Can you work these out from the model? Positions are in its coordinate system, mm. Face numbers are marked on the shaded views. A direction names the side the tool comes from. Give positions to 0.01 mm unless a question says otherwise; leave off trailing zeros. Loops run counter-clockwise (first coordinate to the right, second up) from the corner with the lowest first, then second, coordinate; pieces in that order, holes last. Notation, with made-up numbers: M 1.25,-17 L 17.25,-17 A6 ccw 17.25,-7 Z; hole C -10,44 d4. An arc over 180 degrees is marked long. Answer as a JSON object with one key per item and string values.
Autodesk Inventor part; units mm, degrees
ref_plane "Work Plane1" through (0, 0, 15) normal (0, 0, -1) x (-1, 0, 0)
ref_plane "YZ Plane" through (0, 0, 0) normal (1, 0, 0) x (0, 1, 0)
ref_plane "XZ Plane" through (0, 0, 0) normal (0, 1, 0) x (-1, 0, 0)
sketch "Sketch1" plane through (0, 0, 0) normal (0, 0, 1) x (1, 0, 0)
  line L0 (-12.5, 12.5) -> (12.5, 12.5) construction
  line L1 (12.5, 12.5) -> (12.5, -12.5) construction
  line L2 (12.5, -12.5) -> (-12.5, -12.5) construction
  line L3 (-12.5, -12.5) -> (-12.5, 12.5) construction
  line L4 (-12.5, 12.5) -> (12.5, -12.5) construction
  line L5 (12.5, 12.5) -> (-12.5, -12.5) construction
  circle A0 centre (-12.5, 12.5) radius 3
  circle A1 centre (12.5, 12.5) radius 3
  circle A2 centre (12.5, -12.5) radius 3
  circle A3 centre (-12.5, -12.5) radius 3
  line L6 (-18.5, -18.5) -> (18.5, -18.5)
  line L7 (18.5, -18.5) -> (18.5, -6.5)
  line L8 (18.5, -6.5) -> (-18.5, -6.5)
  line L9 (-18.5, -6.5) -> (-18.5, -18.5)
  line L10 (-18.5, -18.5) -> (18.5, -6.5) construction
  line L11 (18.5, -18.5) -> (-18.5, -6.5) construction
  point P0 (0, 0)
  point P1 (0, -12.5)
  dimension "d0" = 25
  dimension "d1" = 25
  dimension "d2" = 6
  dimension "d3" = 6
  dimension "d4" = 6
  dimension "d5" = 6
  dimension "d38" = 37
  dimension "d39" = 12
extrude "Extrusion8" add sketch "Sketch1" against normal blind 3 contours L9 L8 L7 L6
ref_plane "Work Plane1" through (0, 0, 15) normal (0, 0, -1) x (-1, 0, 0)
sketch "Sketch4" plane through (0, 0, 0) normal (1, 0, 0) x (0, 1, 0)
  line L0 (-6.5, 0) -> (-18.5, 0)
  line L1 (-18.5, 0) -> (-6.5, 0)
  line L2 (-6.5, 0) -> (-6.5, 10)
  line L3 (-6.5, 10) -> (-18.5, 10)
  line L4 (-18.5, 10) -> (-18.5, 0)
  circle A0 centre (-0.5, 26) radius 15
  circle A1 centre (-0.5, 26) radius 18
  line L5 (-18.5, 10) -> (-18.5, 26)
  point P0 (-12.5, 10)
  point P1 (-18.5, 9.0294)
  point P2 (-6.5, 9.0294)
  dimension "d57" = 10
  dimension "d58" = 30
  dimension "d59" = 3
  dimension "d61" = 18
extrude "Extrusion9" add sketch "Sketch4" along normal mid plane 7
properties part number "syringe_mount"
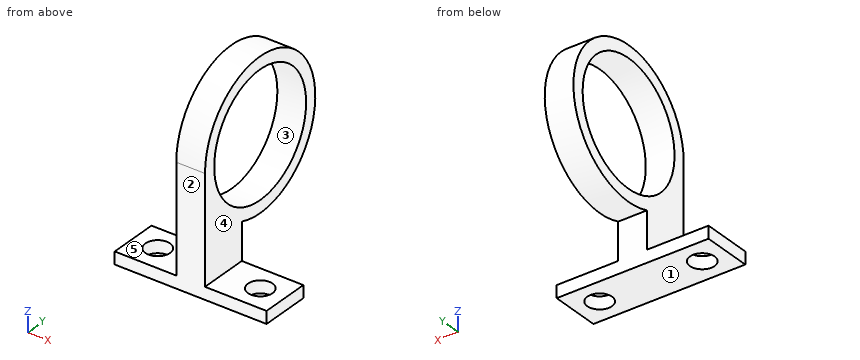
1) Will these pins go through, and if not, where does the flat tip stop? pin 1 Ø11 at (y, z) = (-0.5, 13.5) entering from -X; pin 2 Ø1.5 at (x, z) = (-2, 20) entering from +Y; pin 3 Ø9.5 at (x, y) = (-9, -12.5) entering from +Z.
Answer list:
{"pin 1": "x = -3.5", "pin 2": "y = 16.72", "pin 3": "z = 0"}
2) Suppose I cut it at A-A, the plane y = -0.5. Write out the boundary of the cut face in (x, z).
Answer list:
{"outline": "M -3.5,8 L 3.5,8 L 3.5,11 L -3.5,11 Z; M -3.5,41 L 3.5,41 L 3.5,44 L -3.5,44 Z"}
3) Suppose I cut it at D-D, the plane x = 8.5. Write out the boundary of the cut face in (y, z), and give its area (3 significant figures).
Answer list:
{"outline": "M -18.5,-3 L -6.5,-3 L -6.5,0 L -18.5,0 Z", "area": "36.0 mm^2"}
4) Suppose I cut it at C-C, the plane x = -0.5. Write out the boundary of the cut face in (y, z), and give its area (3 significant figures).
Answer list:
{"outline": "M -18.5,-3 L -6.5,-3 L -6.5,9.03 A18 ccw long -18.5,26 Z; hole C -0.5,26 d30", "area": "511 mm^2"}
5) For the marked faces 4 and 5, which set-ups out of +Z, -Z, +X, -X, +Y, -Y let a thin tool reach every point of the face, with its end or its side?
Answer list:
{"face 4": "+Z, +X, +Y, -Y", "face 5": "+Z, -X, +Y, -Y"}
6) Suppose I cut it at B-B, the plane z = 31. Write out the boundary of the cut face in (x, y), and give its area (3 significant figures).
Answer list:
{"outline": "M -3.5,-17.79 L 3.5,-17.79 L 3.5,-14.64 L -3.5,-14.64 Z; M -3.5,13.64 L 3.5,13.64 L 3.5,16.79 L -3.5,16.79 Z", "area": "44.1 mm^2"}
7) Please list where these lines run through material, in increasing order: line 1 along Z through (x, y) = (2, -0.5); line 2 along Y through (x, z) = (-12.5, -0.75); line 3 along X through (y, z) = (-16, 31.5). Write a range as from..to.
Answer list:
{"line 1": "8..11, 41..44", "line 2": "-18.5..-15.5, -9.5..-6.5", "line 3": "-3.5..3.5"}
8) If we mould it in two halves opening along Y, with no side actions, what happens to the marked faces 1, 2 and 3? For each: +Y half, -Y half, draft (parallel to the pull), parting line (faces both ways), or undercut.
Answer list:
{"face 1": "draft", "face 2": "-Y half", "face 3": "undercut"}
